Can you work these out from the model? Positions are in its coordinate system, mm. Face numbers are marked on the shaded views. A direction names the side the tool comes from. Round coordinates to 2 decimals unless told otherwise and drop trailing zeros. Loops run counter-clockwise (first coordinate to the right, second up) from the corner with the lowest first, then second, coordinate; pieces in that order, holes last. Notation, with made-up numbers: M 30,70.5 L 35,70.5 A15 ccw 35,85.5 Z; hole C -18,3.25 d3. An arc over 180 degrees is marked long. Use a Markdown table: item, result. Add a question column.
```python
from build123d import *

# Parameters (mm, degrees)
SKETCH_1_W        = 40
SKETCH_1_H        = 93
PAD_DEPTH         = 5
PAD_FACE3_W       = 40
PAD_FACE3_H       = 5
PAD011_DEPTH      = 10.2
SKETCH_W          = 40
SKETCH_H          = 7.4
PAD001_DEPTH      = 5
PAD002_DEPTH      = 110.6
SKETCH005_W       = 9.2
SKETCH005_H       = 9.2
POCKET_DEPTH      = 33.001
SKETCH006_W       = 2
SKETCH006_H       = 101.4
PAD006_DEPTH      = 23
SKETCH011_W       = 87.2
SKETCH011_H       = 1.4
PAD010_DEPTH      = 10
PAD012_DEPTH      = 2
PAD013_DEPTH      = 7.2
PAD014_DEPTH      = 2
SKETCH016_W       = 9.2
SKETCH016_H       = 5
PAD015_DEPTH      = 9.2
SKETCH017_R       = 1.6
POCKET001_DEPTH   = 5
SKETCH018_W       = 17.6
SKETCH018_H       = 1.4
PAD016_DEPTH      = 10
SKETCH019_R       = 2
POCKET002_DEPTH   = 2
CHAMFER_SIZE      = 6
CHAMFER001_SIZE   = 2
PAD017_DEPTH      = 1.5
PAD017_DEPTH_BACK = 3
CHAMFER002_SIZE   = 0.99
CHAMFER003_SIZE   = 1


with BuildPart() as part:
    # Sketch_1 → Pad (new body)
    with BuildSketch(Plane.XY):
        with Locations((-20, 46.5)):
            Rectangle(SKETCH_1_W, SKETCH_1_H)
    extrude(amount=PAD_DEPTH)

    # Pad Face3 → Pad011 (add)
    with BuildSketch(Plane(origin=(-20, 93, 2.5), x_dir=(1, 0, 0), z_dir=(0, 1, 0))):
        Rectangle(PAD_FACE3_W, PAD_FACE3_H)
    extrude(amount=PAD011_DEPTH)

    # Sketch → Pad001 (join)
    with BuildSketch(Plane.XY):
        with Locations((-20, -3.7)):
            Rectangle(SKETCH_W, SKETCH_H)
    extrude(amount=PAD001_DEPTH)

    # Sketch001 (on Face9 of Pad001) → Pad002 (join)
    with BuildSketch(Plane.XZ.offset(7.4)):
        Polygon((-40, 5), (-68, -23), (-68, -28), (-66, -28), (-66, -26), (-40, 0), align=None)
    extrude(amount=-PAD002_DEPTH)

    # Sketch005 (on Face11 of Pad002) → Pocket (cut, through all)
    with BuildSketch(Plane.XY.offset(5)):
        with Locations((-63.4, 98.6)):
            Rectangle(SKETCH005_W, SKETCH005_H)
    extrude(amount=-POCKET_DEPTH, mode=Mode.SUBTRACT)

    # Sketch006 → Pad006 (join)
    with BuildSketch(Plane(origin=(0, 0, -28), x_dir=(1, 0, 0), z_dir=(0, 0, -1))):
        with Locations((-67, -43.3)):
            Rectangle(SKETCH006_W, SKETCH006_H)
    extrude(amount=PAD006_DEPTH)

    # Sketch011 → Pad010 (join)
    with BuildSketch(Plane.YZ):
        with Locations((57.4, 2.64)):
            Rectangle(SKETCH011_W, SKETCH011_H)
    extrude(amount=PAD010_DEPTH)

    # Sketch013 (on Face8 of Pad006) → Pad012 (join)
    with BuildSketch(Plane(origin=(0, 103.2, 0), x_dir=(-1, 0, 0), z_dir=(0, 1, 0))):
        Polygon((0, 0), (40, 0), (58.8, -18.8), (58.8, -51), (0, -51), align=None)
    extrude(amount=-PAD012_DEPTH)

    # Sketch014 (on Face24 of Pad012) → Pad013 (join)
    with BuildSketch(Plane.XZ.offset(-101.2)):
        Polygon((-58.8, -51), (-58.8, -18.8), (-56.8, -16.8), (-56.8, -51), (-56.8, -53), (-58.8, -53), align=None)
    extrude(amount=PAD013_DEPTH)

    # Sketch015 (on Face23 of Pad013) → Pad014 (join)
    with BuildSketch(Plane.XZ.offset(-94)):
        Polygon((-56.8, -53), (-66, -53), (-66, -26), (-56.8, -16.8), align=None)
    extrude(amount=PAD014_DEPTH)

    # Sketch016 (on Face41 of Pad014) → Pad015 (join)
    with BuildSketch(Plane(origin=(-58.8, 0, 0), x_dir=(0, -1, 0), z_dir=(-1, 0, 0))):
        with Locations((-98.6, -48.5)):
            Rectangle(SKETCH016_W, SKETCH016_H)
    extrude(amount=PAD015_DEPTH)

    # Sketch017 (on Face49 of Pad015) → Pocket001 (cut)
    with BuildSketch(Plane.XY.offset(-46)):
        with Locations((-62.4, 97.6)):
            Circle(SKETCH017_R)
    extrude(amount=-POCKET001_DEPTH, mode=Mode.SUBTRACT)

    # Sketch018 (on Face12 of Pocket001) → Pad016 (join)
    with BuildSketch(Plane.XZ.offset(7.4)):
        with Locations((-20, 2.64)):
            Rectangle(SKETCH018_W, SKETCH018_H)
    extrude(amount=PAD016_DEPTH)

    # Sketch019 (on Face34 of Pad016) → Pocket002 (cut)
    with BuildSketch(Plane(origin=(0, 103.2, 0), x_dir=(-1, 0, 0), z_dir=(0, 1, 0))):
        with Locations((8, -11)):
            Circle(SKETCH019_R)
        with Locations((8, -43)):
            Circle(SKETCH019_R)
        with Locations((40, -43)):
            Circle(SKETCH019_R)
        with Locations((40, -11)):
            Circle(SKETCH019_R)
        with BuildLine():
            Line((8, -25), (22, -25))
            Line((22, -25), (22, -11))
            ThreePointArc((22, -11), (12.100505, -15.100505), (8, -25))
        make_face()
        with BuildLine():
            Line((26, -25), (26, -11))
            ThreePointArc((40, -25), (35.899495, -15.100505), (26, -11))
            Line((26, -25), (40, -25))
        make_face()
        with BuildLine():
            Line((22, -29), (8, -29))
            ThreePointArc((8, -29), (12.100505, -38.899495), (22, -43))
            Line((22, -29), (22, -43))
        make_face()
        with BuildLine():
            Line((26, -29), (40, -29))
            ThreePointArc((26, -43), (35.899495, -38.899495), (40, -29))
            Line((26, -29), (26, -43))
        make_face()
    extrude(amount=-POCKET002_DEPTH, mode=Mode.SUBTRACT)

    # Chamfer
    chamfer_edges = [part.edges().sort_by_distance(p)[0] for p in [
        (-22, 102.2, -25),
        (-26, 102.2, -25),
        (-22, 102.2, -29),
        (-26, 102.2, -29),
    ]]
    chamfer(chamfer_edges, length=CHAMFER_SIZE)

    # Chamfer001
    chamfer001_edges = [part.edges().sort_by_distance(p)[0] for p in [
        (-20, 103.2, 5),
    ]]
    chamfer(chamfer001_edges, length=CHAMFER001_SIZE)

    # Sketch020 (on Face62 of Chamfer001) → Pad017 (join, two sides)
    with BuildSketch(Plane.XZ.offset(7.4)) as pad017_sk:
        Polygon((-66, -51), (-66, -26), (-65, -25), (-65, -51), align=None)
    extrude(amount=PAD017_DEPTH)
    extrude(pad017_sk.sketch, amount=-PAD017_DEPTH_BACK)

    # Chamfer002
    chamfer002_edges = [part.edges().sort_by_distance(p)[0] for p in [
        (-65, -4.4, -38),
    ]]
    chamfer(chamfer002_edges, length=CHAMFER002_SIZE)

    # Chamfer003
    chamfer003_edges = [part.edges().sort_by_distance(p)[0] for p in [
        (-8, 102.2, -25),
        (-8, 102.2, -29),
        (-22, 102.2, -11),
        (-26, 102.2, -11),
        (-40, 102.2, -25),
        (-40, 102.2, -29),
        (-26, 102.2, -43),
        (-22, 102.2, -43),
    ]]
    chamfer(chamfer003_edges, length=CHAMFER003_SIZE)


solid = part.part
```
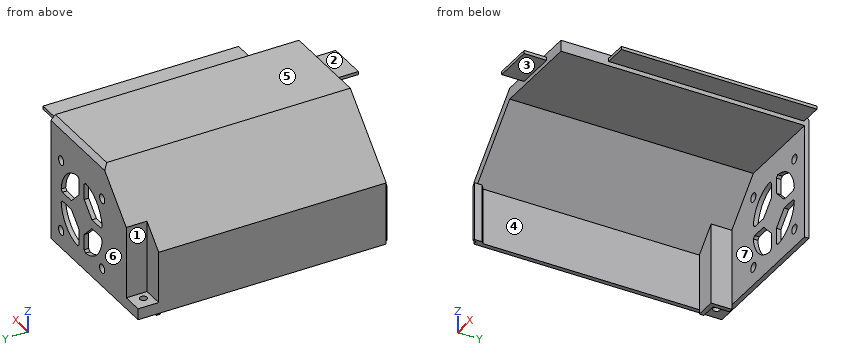
(1) Suppose I cut it at D-D on z = -32. Count the separate pieces of the cut face and the enclosed holes in it, and give its area (3 significant figures).
(2) On a 3-axis mill with a long thin cutter (end or side, diameter ignored), from which of +Z, -Z, +X, -X, +Y, -Y can I reach the whole of each face in a straight line? I mean the marked faces 1, 2 and 3. Say none if no direction works.
(3) If I drill on probe 1 along Y at (x, z) = (-4.5, -7); probe 2 along X at (y, z) = (97.5, -39.5); probe 3 along Z at (x, y) = (-40, 102.55), over which ranges is the centre line in solid material (lowest first)? Write a range as [from, to].
(4) Thinking about a two-plate mould opening in Y: for the marked faces 4, 5, 6 and 7, which applies, released by +Y, released by -Y, zero draft, split by the parting line, or undercut?
(5) Suppose I cut it at A-A on y = 97.6. List the corners of the cut face in (x, z) for me.
(6) Suppose I cut it at B-B on x = -62.4. List the corners of the cut face in (y, z) for me, and give its area (3 significant figures).
(7) Suppose I cut it at C-C on y = 17. List the corners of the cut face in (x, z) for me.
(8) I'm going to push flat-ended pins straight in: pin 1 (1 mm diameter, centred on x = -10, y = 50, fed in from -Z); pin 2 (4.5 mm diameter, centred on x = -62.5, z = -30, fed in from +Y); pin 3 (2 mm diameter, centred on x = -11.5, y = 102.5, fed in from +Z); pin 4 (3 mm diameter, centred on x = -8, z = -43, fed in from +Y). Where does each tip first touch, or does it pass through?
Results below:
| question | item | result |
|---|---|---|
| 1 | separate pieces | 3 |
| 1 | enclosed holes | 0 |
| 1 | area | 315 mm² |
| 2 | face 1 | +Z, -X, +Y |
| 2 | face 2 | +Z, +X, -X, -Y |
| 2 | face 3 | -Z, +X, -X, -Y |
| 3 | probe 1 | y = [101.2, 103.2] |
| 3 | probe 2 | x = [-58.8, -56.8] |
| 3 | probe 3 | z = [-51, -45], [-41, -13], [-9, 3.65] |
| 4 | face 4 | undercut |
| 4 | face 5 | zero draft |
| 4 | face 6 | released by +Y |
| 4 | face 7 | released by -Y |
| 5 | outline | M -68,-51 L -64,-51 L -64,-46 L -68,-46 Z; M -60.8,-51 L -58.8,-51 L -58.8,-53 L -56.8,-53 L -56.8,-16.8 L -40,0 L 0,0 L 0,1.94 L 10,1.94 L 10,3.34 L 0,3.34 L 0,5 L -40,5 L -58.8,-13.8 L -58.8,-46 L -60.8,-46 Z |
| 6 | outline | M -7.4,-22.4 L 92,-22.4 L 92,-53 L 94,-53 L 94,-51 L 96,-51 L 96,-46 L 94,-46 L 94,-17.4 L -7.4,-17.4 Z; M 99.2,-51 L 103.2,-51 L 103.2,-46 L 99.2,-46 Z |
| 6 | area | 598 mm² |
| 7 | outline | M -68,-51 L -66,-51 L -66,-26 L -40,0 L 0,0 L 0,1.94 L 10,1.94 L 10,3.34 L 0,3.34 L 0,5 L -40,5 L -68,-23 Z |
| 8 | pin 1 | stops at z = 0 |
| 8 | pin 2 | stops at y = 94 |
| 8 | pin 3 | stops at z = 4.7 |
| 8 | pin 4 | passes through |
